Autodesk Inventor part; units mm, degrees
ref_plane "YZ Plane" through (0, 0, 0) normal (1, 0, 0) x (0, 1, 0)
ref_plane "XZ Plane" through (0, 0, 0) normal (0, 1, 0) x (-1, 0, 0)
ref_plane "XY Plane" through (0, 0, 0) normal (0, 0, 1) x (1, 0, 0)
sketch "Sketch3" plane through (0, 0, 0) normal (0, 0, 1) x (1, 0, 0)
  line L0 (-23.255, 22.635) -> (-23.255, -9.435)
  line L1 (-18.255, -32.435) -> (-8.145, -32.435)
  line L2 (-8.145, -32.435) -> (-8.145, -29.435)
  line L3 (-8.145, -29.435) -> (-20.255, -29.435)
  line L4 (-20.255, -29.435) -> (-20.255, 42.635)
  line L5 (-20.255, 42.635) -> (-8.145, 42.635)
  line L6 (-8.145, 42.635) -> (-8.145, 45.635)
  line L7 (-8.145, 45.635) -> (-18.255, 45.635)
  arc A0 (-23.255, 40.635) -> (-23.255, 22.635) centre (-23.255, 31.635) ccw
  circle A1 centre (-27.755, 31.635) radius 1.25
  line L8 (-8.145, 45.635) -> (-18.255, 45.635)
  line L9 (-18.255, -32.435) -> (-8.145, -32.435)
  line L10 (-8.145, -29.435) -> (7.855, -29.435)
  line L11 (-8.145, -32.435) -> (-8.145, -29.435)
  line L12 (7.855, -32.435) -> (-8.145, -32.435)
  line L13 (7.855, -32.435) -> (7.855, -29.435)
  line L14 (7.855, 42.635) -> (-8.145, 42.635)
  line L15 (7.855, 45.635) -> (7.855, 42.635)
  line L16 (-8.145, 45.635) -> (7.855, 45.635)
  line L17 (-8.145, 45.635) -> (-8.145, 42.635)
  line L18 (-23.255, 22.635) -> (-23.255, -9.435)
  arc A2 (-23.255, -27.435) -> (-18.255, -32.435) centre (-18.255, -27.435) ccw
  line L19 (-8.145, -32.435) -> (-8.145, -29.435)
  line L20 (-8.145, -29.435) -> (-20.255, -29.435)
  line L21 (-20.255, -29.435) -> (-20.255, 42.635)
  line L22 (-20.255, 42.635) -> (-8.145, 42.635)
  line L23 (-8.145, 42.635) -> (-8.145, 45.635)
  arc A3 (-18.255, 45.635) -> (-23.255, 40.635) centre (-18.255, 40.635) ccw
  arc A4 (-23.255, 40.635) -> (-23.255, 22.635) centre (-23.255, 31.635) ccw
  circle A5 centre (-27.755, 31.635) radius 1.25
  arc A6 (-23.255, -27.435) -> (-18.255, -32.435) centre (-18.255, -27.435) ccw
  arc A7 (-18.255, 45.635) -> (-23.255, 40.635) centre (-18.255, 40.635) ccw
  line L24 (40.455, -9.435) -> (40.455, 22.635)
  arc A8 (40.455, 40.635) -> (35.455, 45.635) centre (35.455, 40.635) ccw
  line L25 (35.455, 45.635) -> (7.855, 45.635)
  line L26 (7.855, 45.635) -> (7.855, 42.635)
  line L27 (7.855, 42.635) -> (37.455, 42.635)
  line L28 (37.455, 42.635) -> (37.455, -29.435)
  line L29 (37.455, -29.435) -> (7.855, -29.435)
  line L30 (7.855, -29.435) -> (7.855, -32.435)
  line L31 (7.855, -32.435) -> (35.455, -32.435)
  arc A9 (35.455, -32.435) -> (40.455, -27.435) centre (35.455, -27.435) ccw
  arc A10 (40.455, -27.435) -> (40.455, -9.435) centre (40.455, -18.435) ccw
  circle A11 centre (44.955, -18.435) radius 1.25
  circle A12 centre (-27.755, -18.435) radius 1.25
  arc A13 (-23.255, -9.435) -> (-23.255, -27.435) centre (-23.255, -18.435) ccw
  circle A14 centre (-27.755, -18.435) radius 1.25
  arc A15 (-23.255, -9.435) -> (-23.255, -27.435) centre (-23.255, -18.435) ccw
  circle A16 centre (44.955, 31.635) radius 1.25
  arc A17 (40.455, 22.635) -> (40.455, 40.635) centre (40.455, 31.635) ccw
  point P0 (0, 0)
extrude "Extrusion3" add sketch "Sketch3" along normal blind 3
sketch "Sketch5" plane through (0, 0, 0) normal (0, 0, -1) x (-1, 0, 0)
  line L0 (20.255, -29.435) -> (20.255, 42.635)
  line L1 (8.145, -29.435) -> (20.255, -29.435)
  line L2 (-37.455, -29.435) -> (-7.855, -29.435)
  line L3 (-37.455, 42.635) -> (-37.455, -29.435)
  line L4 (-7.855, 42.635) -> (-37.455, 42.635)
  line L5 (20.255, 42.635) -> (8.145, 42.635)
  line L6 (-7.855, 42.635) -> (8.145, 42.635)
  line L7 (-7.855, -29.435) -> (8.145, -29.435)
  line L8 (20.055, -29.235) -> (-37.255, -29.235)
  line L9 (-37.255, -29.235) -> (-37.255, 42.435)
  line L10 (-37.255, 42.435) -> (-7.855, 42.435)
  line L11 (-7.855, 42.435) -> (8.145, 42.435)
  line L12 (8.145, 42.435) -> (20.055, 42.435)
  line L13 (20.055, 42.435) -> (20.055, -29.235)
  line L14 (-36.255, -28.235) -> (19.055, -28.235)
  line L15 (19.055, -28.235) -> (19.055, 41.435)
  line L16 (19.055, 41.435) -> (-36.255, 41.435)
  line L17 (-36.255, 41.435) -> (-36.255, -28.235)
  point P0 (0, 0)
  dimension "d8" = 0.2
  dimension "d9" = 1
extrude "Extrusion4" add sketch "Sketch5" along normal blind 2 contours L8 L9 L10 L11 L12 L13
properties part number "lid_arm"
Here's how the part is built. I have some questions about the finished solid (model axes, mm). A direction names the side the tool comes from. Give positions to 0.01 mm unless a question says otherwise; leave off trailing zeros. Write each loop counter-clockwise with the first axis right and the second up, starting at its lowest first coordinate (ties: lowest second). Pieces come first, ordered by that corner, then holes. Notation, with made-up numbers: M -33,69 L -6,69 A24 ccw -6,107 Z; hole C -32.75,18.25 d1. An arc over 180 degrees is marked long. Put each result on its own line as item: value. Start each with the question number.
Item 1: If we section it at C-C, the plane y = 39: Write out the boundary of the cut face in (x, z) (3 decimals), then the cut area to 3 significant figures.
Item 2: On a 3-axis mill with a long thin cutter (end or side, diameter ignored), from which of +Z, -Z, +X, -X, +Y, -Y can I reach the whole of each face in a straight line? I mean faces 4 (the flat face through (9, 42.435, -1)), 5 (the flat face through (37.255, 6, -1)), 6 (the flat face through (8, 7, 0)), 7 (the flat face through (-23.255, 7, 1)). Say none if no direction works.
Item 3: Will these pins go through, and if not, where does the flat tip stop? pin 1 (2 mm diameter, centred on x = 44.955, y = 31.635, fed in from +Z); pin 2 (1.5 mm diameter, centred on y = 2.5, z = 1, fed in from +X) (3 decimals); pin 3 (6 mm diameter, centred on x = 29, y = 4.5, fed in from -Z); pin 4 (1 mm diameter, centred on x = 17, z = -1.5, fed in from +Y) (3 decimals).
Item 4: If we section it at B-B, the plane z = -0.95: Write out the boundary of the cut face in (x, y) (3 decimals), then the cut area to 3 significant figures.
Item 5: If we section it at A-A, the plane x = 27.5: Write out the boundary of the cut face in (y, z) (3 decimals), then the cut area to 3 significant figures.
Item 6: I need wall thicknesses on L1, parallel to Y at x = -23.5, z = 1; L2, parallel to X at y = -18, z = 2.85; L3, parallel to X at y = -24, z = -1.2 (3 decimals). Which ranges of each line are inside material? Lowest first, please. Write a range as from..to.
Item 7: Thinking about a two-plate mould opening in X: for faces 1 (the cylindrical face through (-21.83, 44.13, 1.48)), 2 (the flat face through (9, 45.635, 1)), 3 (the cylindrical face through (43.706, -18.49, 1.479)), which applies, +X half, -X half, draft (parallel to the pull), parting line (faces both ways), or undercut?
Item 8: If we section it at D-D, the plane x = 42: Write out the boundary of the cut face in (y, z).
Values:
1. outline: M -28.428,0 L -20.055,0 L -20.055,-2 L -19.055,-2 L -19.055,0 L 36.255,0 L 36.255,-2 L 37.255,-2 L 37.255,0 L 45.628,0 L 45.628,3 L -28.428,3 Z
1. area: 226 mm²
2. face 4: -Z, +X, -X, +Y
2. face 5: -Z, +X, +Y, -Y
2. face 6: -Z
2. face 7: +Z, -Z, -X
3. pin 1: through
3. pin 2: x = 40.455
3. pin 3: z = 0
3. pin 4: y = 42.435
4. outline: M -20.055,-29.235 L 37.255,-29.235 L 37.255,42.435 L -20.055,42.435 Z; hole M -19.055,-28.235 L 36.255,-28.235 L 36.255,41.435 L -19.055,41.435 Z
4. area: 254 mm²
5. outline: M -32.435,0 L -29.235,0 L -29.235,-2 L -28.235,-2 L -28.235,0 L 41.435,0 L 41.435,-2 L 42.435,-2 L 42.435,0 L 45.635,0 L 45.635,3 L -32.435,3 Z
5. area: 238 mm²
6. L1: -27.43..-9.44, 22.64..40.63
6. L2: -32.24..-28.93, -26.58..43.78, 46.13..49.44
6. L3: -20.055..-19.055, 36.255..37.255
7. face 1: -X half
7. face 2: draft
7. face 3: undercut
8. outline: M -27.3,0 L -9.57,0 L -9.57,3 L -27.3,3 Z; M 22.77,0 L 40.5,0 L 40.5,3 L 22.77,3 Z
